Design review of the part built by this model. Coordinates are the model's own, in mm. Face numbers are marked on the shaded views. Coordinates: 2 decimals unless noted, no trailing zeros. Loops run counter-clockwise (first coordinate to the right, second up) from the corner with the lowest first, then second, coordinate; pieces in that order, holes last. Notation, with made-up numbers: (86.25, -38.75) - (105.25, -38.75) arc R11 cw to (105.25, -34.75) - close; hole circle Ø3 at (-17, 81). An arc over 180 degrees is marked (long way). One line per question, with ' | ' between items.
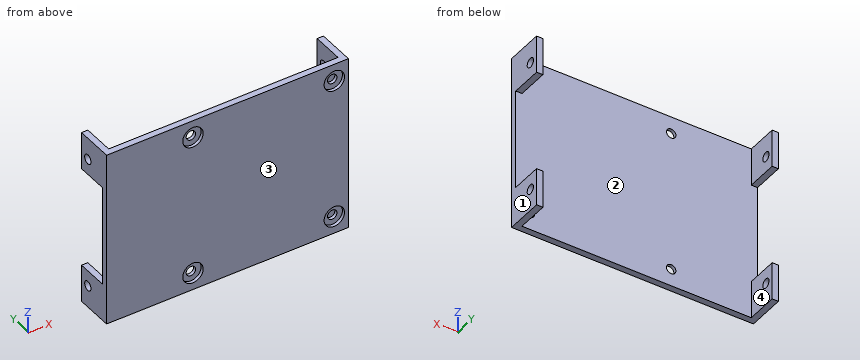
from build123d import *

# Parameters (mm, degrees)
SKETCH1_W           = 77
SKETCH1_H           = 56
BOSS_EXTRUDE1_DEPTH = 2
SKETCH2_R           = 1.5
CUT_EXTRUDE1_DEPTH  = 3
SKETCH3_W           = 2
SKETCH3_H           = 12
BOSS_EXTRUDE2_DEPTH = 10
SKETCH4_R           = 1.5
CUT_EXTRUDE2_DEPTH  = 78
SKETCH5_R           = 3.25
CUT_EXTRUDE3_DEPTH  = 1


with BuildPart() as part:
    # Sketch1 → Boss-Extrude1 (new body)
    with BuildSketch(Plane(origin=(0, 0, 0), x_dir=(1, 0, 0), z_dir=(0, 1, 0))):
        with Locations((-3.12052506, -6.090692124)):
            Rectangle(SKETCH1_W, SKETCH1_H)
    extrude(amount=BOSS_EXTRUDE1_DEPTH)

    # Sketch2 → Cut-Extrude1 (cut, through all)
    with BuildSketch(Plane(origin=(0, 2, 0), x_dir=(1, 0, 0), z_dir=(0, 1, 0))):
        with Locations((30.87947494, 16.409307876)):
            Circle(SKETCH2_R)
        with Locations((30.87947494, -28.590692124)):
            Circle(SKETCH2_R)
        with Locations((-14.12052506, 16.409307876)):
            Circle(SKETCH2_R)
        with Locations((-14.12052506, -28.590692124)):
            Circle(SKETCH2_R)
    extrude(amount=-CUT_EXTRUDE1_DEPTH, mode=Mode.SUBTRACT)

    # Sketch3 → Boss-Extrude2 (add)
    with BuildSketch(Plane(origin=(0, 2, 0), x_dir=(1, 0, 0), z_dir=(0, 1, 0))):
        with Locations((34.37947494, 15.909307876)):
            Rectangle(SKETCH3_W, SKETCH3_H)
        with Locations((34.37947494, -28.090692124)):
            Rectangle(SKETCH3_W, SKETCH3_H)
        with Locations((-40.62052506, 15.909307876)):
            Rectangle(SKETCH3_W, SKETCH3_H)
        with Locations((-40.62052506, -28.090692124)):
            Rectangle(SKETCH3_W, SKETCH3_H)
    extrude(amount=BOSS_EXTRUDE2_DEPTH)

    # Sketch4 → Cut-Extrude2 (cut, through all)
    with BuildSketch(Plane(origin=(35.37947494, 0, 0), x_dir=(0, 0, -1), z_dir=(1, 0, 0))):
        with Locations((-27.090692124, 9)):
            Circle(SKETCH4_R)
        with Locations((14.909307876, 9)):
            Circle(SKETCH4_R)
    extrude(amount=-CUT_EXTRUDE2_DEPTH, mode=Mode.SUBTRACT)

    # Sketch5 → Cut-Extrude3 (cut)
    with BuildSketch(Plane(origin=(0, 0, 0), x_dir=(-1, 0, 0), z_dir=(0, -1, 0))):
        with Locations((14.12052506, -28.590692124)):
            Circle(SKETCH5_R)
        with Locations((-30.87947494, -28.590692124)):
            Circle(SKETCH5_R)
        with Locations((-30.87947494, 16.409307876)):
            Circle(SKETCH5_R)
        with Locations((14.12052506, 16.409307876)):
            Circle(SKETCH5_R)
    extrude(amount=-CUT_EXTRUDE3_DEPTH, mode=Mode.SUBTRACT)


solid = part.part
Q1. Take a section at D-D (x = -14.5). Give the boundary of the cut face in (y, z), plus the area to 3 significant figures.
Returned:
outline: (0, -21.91) - (2, -21.91) - (2, -17.86) - (1, -17.86) - (1, -19.64) - (0, -19.64) - close; (0, -13.18) - (1, -13.18) - (1, -14.96) - (2, -14.96) - (2, 27.14) - (1, 27.14) - (1, 25.36) - (0, 25.36) - close; (0, 31.82) - (1, 31.82) - (1, 30.04) - (2, 30.04) - (2, 34.09) - (0, 34.09) - close | area: 93.3 mm²
Q2. Take a section at A-A (y = 3). Give the boundary of the cut face in (x, z).
Returned:
outline: (-41.62, -21.91) - (-39.62, -21.91) - (-39.62, -9.91) - (-41.62, -9.91) - close; (-41.62, 22.09) - (-39.62, 22.09) - (-39.62, 34.09) - (-41.62, 34.09) - close; (33.38, -21.91) - (35.38, -21.91) - (35.38, -9.91) - (33.38, -9.91) - close; (33.38, 22.09) - (35.38, 22.09) - (35.38, 34.09) - (33.38, 34.09) - close
Q3. To check wall thickness, follow line 1 along X through (y, z) = (2.25, 24); line 2 along Y through (x, z) = (-3.5, -1). State the ranges of each line that lie inside material, in increasing order.
Returned:
line 1: x = -41.62 to -39.62, 33.38 to 35.38 | line 2: y = 0 to 2
Q4. Take a section at B-B (z = 24.5). Give the boundary of the cut face in (x, y), plus the area to 3 significant figures.
Returned:
outline: (-41.62, 0) - (35.38, 0) - (35.38, 12) - (33.38, 12) - (33.38, 2) - (-39.62, 2) - (-39.62, 12) - (-41.62, 12) - close | area: 194 mm²
Q5. Draft analysis for pull direction X (two halves, no side actions). For the marked faces 1, 2, 3 and 4, state which applies: +X half, -X half, draft (parallel to the pull), parting line (faces both ways), or undercut.
Returned:
face 1: +X half | face 2: undercut | face 3: draft | face 4: undercut
Q6. Take a section at C-C (y = 9). State how many separate pieces and enclosed holes the cut face has, plus the area to 3 significant figures.
Returned:
separate pieces: 8 | enclosed holes: 0 | area: 72.0 mm²
Q7. For pin 1 (17 mm diameter, centred on x = -2, z = -4, fed in from +Y); pin 2 (3.5 mm diameter, centred on x = -14.12, z = 28.59, fed in from -Y), all flat-tipped, find the tip position at first contact; note any pin that passes through.
Returned:
pin 1: stops at y = 2 | pin 2: stops at y = 1
